from build123d import *


with BuildPart() as part:
    # Эскиз1 → Повернуть1 (revolve)
    with BuildSketch(Plane.XY, mode=Mode.PRIVATE) as revolve_1_sk:
        with BuildLine():
            Line((-92.36476601, 115), (-48, 115))
            ThreePointArc((-48, 115), (-45.878679656, 115.878679656), (-45, 118))
            Line((-45, 118), (-45, 164))
            Line((-45, 164), (-40, 164))
            Line((-40, 164), (-40, 276))
            Line((-40, 276), (-38, 278))
            Line((-38, 278), (0, 278))
            Line((0, 278), (0, -224))
            Line((0, -224), (-38, -224))
            Line((-38, -224), (-40, -222))
            Line((-40, -222), (-40, -164))
            Line((-40, -164), (-45, -164))
            Line((-45, -164), (-45, -118))
            ThreePointArc((-45, -118), (-45.878679656, -115.878679656), (-48, -115))
            Line((-48, -115), (-92.36476601, -115))
            ThreePointArc((-92.36476601, -115), (-147.5, 0), (-92.36476601, 115))
        make_face()
    revolve(revolve_1_sk.sketch.rotate(Axis((0, 332.383276995, 0), (0, -1, 0)), 270), axis=Axis((0, 332.383276995, 0), (0, -1, 0)))


solid = part.part
The listing builds one solid part. Answer for the finished solid, in the listing's coordinates (mm). A direction names the side the tool comes from. Give positions to 0.01 mm unless a question says otherwise; leave off trailing zeros. Write each loop counter-clockwise with the first axis right and the second up, starting at its lowest first coordinate (ties: lowest second). Pieces come first, ordered by that corner, then holes.
1) Section B-B (z = 0) is taken. Write down the section's boundary in (x, y).
2) Section D-D (z = 109) is taken. Write down the section's boundary in (x, y).
3) Given P1, Ø2, axis at y = -104.5, z = 47, coming from the -X side; P2, Ø3, axis at x = -60.5, y = 14.5, coming from the -Z side; P3, Ø1, axis at y = 60.5, z = -57, coming from the +X side, each flat-ended and moving along its own axis, determine where each tip first touches the part or whether it passes through.
4) Section C-C (y = 147) is taken. Write down the section's boundary in (x, z).
5) Section A-A (x = 0) is taken. Write down the section's boundary in (y, z).
6) Find the intervals of material crossed by L1, parallel to Y at x = 65.5, z = -57; L2, parallel to Y at x = -92.5, z = -15.5; L3, parallel to X at y = 21, z = -107, in increasing order.
7) A tool of negligible diameter and unlimited length cuts with its end or side. For faces 1 (the face through (26.5, -164, 30.2)), 2 (the face through (39.05, 220.78, -8.67)), 3 (the face through (-1, 278, -1)), from which of +Z, -Z, +X, -X, +Y, -Y can it reach the whole face along a straight path? Write none if from no direction.
Response:
1. outline: (-92.36, -115) - (-48, -115) arc R3 cw to (-45, -118) - (-45, -164) - (-40, -164) - (-40, -222) - (-38, -224) - (38, -224) - (40, -222) - (40, -164) - (45, -164) - (45, -118) arc R3 cw to (48, -115) - (92.36, -115) arc R147.5 ccw to (92.36, 115) - (48, 115) arc R3 cw to (45, 118) - (45, 164) - (40, 164) - (40, 276) - (38, 278) - (-38, 278) - (-40, 276) - (-40, 164) - (-45, 164) - (-45, 118) arc R3 cw to (-48, 115) - (-92.36, 115) arc R147.5 ccw to start
2. outline: circle Ø198.75 at (0, 0)
3. P1: stops at x = -94.1
3. P2: stops at z = -134.43
3. P3: stops at x = 122.19
4. outline: circle Ø90 at (0, 0)
5. outline: (-224, -38) - (-222, -40) - (-164, -40) - (-164, -45) - (-118, -45) arc R3 cw to (-115, -48) - (-115, -92.36) arc R147.5 ccw to (115, -92.36) - (115, -48) arc R3 cw to (118, -45) - (164, -45) - (164, -40) - (276, -40) - (278, -38) - (278, 38) - (276, 40) - (164, 40) - (164, 45) - (118, 45) arc R3 cw to (115, 48) - (115, 92.36) arc R147.5 ccw to (-115, 92.36) - (-115, 48) arc R3 cw to (-118, 45) - (-164, 45) - (-164, 40) - (-222, 40) - (-224, 38) - close
6. L1: y = -115 to 115
6. L2: y = -113.84 to 113.84
6. L3: x = -99.33 to 99.33
7. face 1: -Y
7. face 2: +Y
7. face 3: +Z, -Z, +X, -X, +Y
